from build123d import *

# Parameters (mm, degrees)
SKETCH_1_R          = 1.25
EXTRUDE_1_DEPTH     = 5
SKETCH_2_W          = 2.5
SKETCH_2_H          = 30.5
EXTRUDE_2_DEPTH     = 22.5
CUT_EXTRUDE_1_REACH = 107
SKETCH_4_R          = 3.5
SKETCH_4_R_2        = 1.25
SKETCH_4_W          = 30.5
SKETCH_4_H          = 14.5
EXTRUDE_3_DEPTH     = 2


with BuildPart() as part:
    # Эскиз1 → Бобышка-Вытянуть1 (new body)
    with BuildSketch(Plane(origin=(0, 0, 0), x_dir=(1, 0, 0), z_dir=(0, 1, 0))):
        with BuildLine():
            Line((-50, 32.5), (50, 32.5))
            ThreePointArc((50, 32.5), (51.767766953, 31.767766953), (52.5, 30))
            Line((52.5, 30), (52.5, -30))
            ThreePointArc((52.5, -30), (51.767766953, -31.767766953), (50, -32.5))
            Line((50, -32.5), (-50, -32.5))
            ThreePointArc((-50, -32.5), (-51.767766953, -31.767766953), (-52.5, -30))
            Line((-52.5, -30), (-52.5, -27.5))
            Line((-52.5, -27.5), (-52.5, 27.5))
            Line((-52.5, 27.5), (-52.5, 30))
            ThreePointArc((-52.5, 30), (-51.767766953, 31.767766953), (-50, 32.5))
        make_face()
        with Locations((-47.144457485, 27.207649218)):
            Circle(SKETCH_1_R, mode=Mode.SUBTRACT)
        with Locations((47.144457485, -27.207649218)):
            Circle(SKETCH_1_R, mode=Mode.SUBTRACT)
        with Locations((47.144457485, 27.207649218)):
            Circle(SKETCH_1_R, mode=Mode.SUBTRACT)
        with Locations((-47.144457485, -27.207649218)):
            Circle(SKETCH_1_R, mode=Mode.SUBTRACT)
        with BuildLine():
            Line((-40.944886513, 30), (40.944886513, 30))
            ThreePointArc((40.944886513, 30), (42.446070129, 29.321532349), (42.928749224, 27.74644775))
            ThreePointArc((42.928749224, 27.74644775), (44.154618836, 24.187158388), (47.726226395, 22.997655757))
            ThreePointArc((47.726226395, 22.997655757), (49.313859351, 22.524386076), (50, 21.016482364))
            Line((50, 21.016482364), (50, -21.016482364))
            ThreePointArc((50, -21.016482364), (49.313859351, -22.524386076), (47.726226395, -22.997655757))
            ThreePointArc((47.726226395, -22.997655757), (44.154618836, -24.187158388), (42.928749224, -27.74644775))
            ThreePointArc((42.928749224, -27.74644775), (42.446070129, -29.321532349), (40.944886513, -30))
            Line((40.944886513, -30), (-40.944886513, -30))
            ThreePointArc((-40.944886513, -30), (-42.446070129, -29.321532349), (-42.928749224, -27.74644775))
            ThreePointArc((-42.928749224, -27.74644775), (-44.154618836, -24.187158388), (-47.726226395, -22.997655757))
            ThreePointArc((-47.726226395, -22.997655757), (-49.313859351, -22.524386076), (-50, -21.016482364))
            Line((-50, -21.016482364), (-50, 21.016482364))
            ThreePointArc((-50, 21.016482364), (-49.313859351, 22.524386076), (-47.726226395, 22.997655757))
            ThreePointArc((-47.726226395, 22.997655757), (-44.154618836, 24.187158388), (-42.928749224, 27.74644775))
            ThreePointArc((-42.928749224, 27.74644775), (-42.446070129, 29.321532349), (-40.944886513, 30))
        make_face(mode=Mode.SUBTRACT)
    extrude(amount=EXTRUDE_1_DEPTH)

    # Эскиз2 → Бобышка-Вытянуть2 (add)
    with BuildSketch(Plane.XZ):
        with Locations((-51.25, 0)):
            Rectangle(SKETCH_2_W, SKETCH_2_H)
    extrude(amount=EXTRUDE_2_DEPTH)

    # Эскиз3 → Вырез-Вытянуть1 (cut, up to next)
    with BuildSketch(Plane.ZY.offset(52.5), mode=Mode.PRIVATE) as cut_extrude_1_sk1:
        with BuildLine():
            Line((-15.25, -22.5), (15.25, -22.5))
            ThreePointArc((15.25, -22.5), (0, -7.25), (-15.25, -22.5))
        make_face()
    cut_extrude_1_tool1 = extrude(cut_extrude_1_sk1.sketch, amount=-CUT_EXTRUDE_1_REACH, mode=Mode.PRIVATE) & part.part
    add(cut_extrude_1_tool1.solids().sort_by_distance((-52.5, -16.027699, 0))[0], mode=Mode.SUBTRACT)

    # Эскиз4 → Бобышка-Вытянуть3 (add)
    with BuildSketch(Plane(origin=(0, 5, 0), x_dir=(1, 0, 0), z_dir=(0, 1, 0))):
        with BuildLine():
            Line((-49.4756814, 32.562921498), (49.4756814, 32.562921498))
            ThreePointArc((49.4756814, 32.562921498), (51.597001743, 31.684241842), (52.4756814, 29.562921498))
            Line((52.4756814, 29.562921498), (52.4756814, -29.509131029))
            ThreePointArc((52.4756814, -29.509131029), (51.597001743, -31.630451373), (49.4756814, -32.509131029))
            Line((49.4756814, -32.509131029), (-49.4756814, -32.509131029))
            ThreePointArc((-49.4756814, -32.509131029), (-51.597001743, -31.630451373), (-52.4756814, -29.509131029))
            Line((-52.4756814, -29.509131029), (-52.4756814, 29.562921498))
            ThreePointArc((-52.4756814, 29.562921498), (-51.597001743, 31.684241842), (-49.4756814, 32.562921498))
        make_face()
        with Locations((26.75, -20)):
            Circle(SKETCH_4_R, mode=Mode.SUBTRACT)
        with Locations((-47.144457485, 27.207649218)):
            Circle(SKETCH_4_R_2, mode=Mode.SUBTRACT)
        with Locations((47.144457485, 27.207649218)):
            Circle(SKETCH_4_R_2, mode=Mode.SUBTRACT)
        with Locations((47.144457485, -27.207649218)):
            Circle(SKETCH_4_R_2, mode=Mode.SUBTRACT)
        with Locations((-47.144457485, -27.207649218)):
            Circle(SKETCH_4_R_2, mode=Mode.SUBTRACT)
        with Locations((26.75, 4.25)):
            Rectangle(SKETCH_4_W, SKETCH_4_H, mode=Mode.SUBTRACT)
    extrude(amount=EXTRUDE_3_DEPTH)


solid = part.part
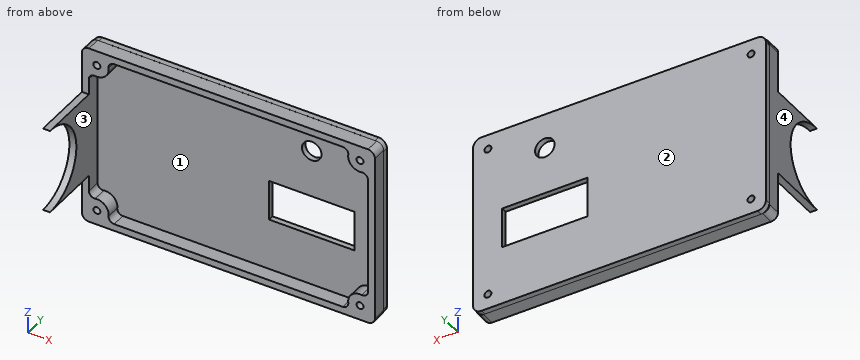
Source: CAD feature listing. Evaluate the final solid. Frame: model axes, mm. Face numbers are marked on the shaded views. A direction names the side the tool comes from. Give positions to 0.01 mm unless a question says otherwise; leave off trailing zeros. Write each loop counter-clockwise with the first axis right and the second up, starting at its lowest first coordinate (ties: lowest second). Pieces come first, ordered by that corner, then holes. Notation, with made-up numbers: M -16,28.25 L -4,28.25 A15 ccw -4,35.25 Z; hole C -25.5,-17 d5. An arc over 180 degrees is marked long. Return JSON: item names as keys, results as strings. Group by question number.
1) Set-up query: the marked faces 1 and 2. Return all of +Z, -Z, +X, -X, +Y, -Y with unobstructed straight access to the full face (end or side cutting, diameter ignored); none if empty.
2) First-contact query: pin 1 Ø2.5 at (x, y) = (10, 2.5) entering from -Z; pin 2 Ø1.6 at (y, z) = (6, 14) entering from -X; pin 3 Ø12 at (x, z) = (17, 15.5) entering from -Y; pin 4 Ø1.5 at (x, z) = (-47.14, 27.21) entering from -Y. Flat tips, straight axial feed; report the tip coordinate or a pass-through.
3) Cut plane C-C, the plane y = -11.25. Output: boundary loops of the cut face in (x, z), then the cut area to 3 significant figures.
4) Ray query, L1, parallel to Z at x = 14, y = 4.25; L2, parallel to X at y = 3.5, z = -17; L3, parallel to Y at x = -43.5, z = -19.5. Return the intervals inside material, ascending.
5) Draft query along Z for the marked faces 3 and 4. Return one class per face: released by +Z, released by -Z, zero draft, split by the parting line, or undercut.
Data:
{
 "1": {"face 1": "-Y", "face 2": "+Z, -Z, +X, -X, +Y"},
 "2": {"pin 1": "stops at z = -32.5", "pin 2": "stops at x = -52.48", "pin 3": "stops at y = 5", "pin 4": "passes through"},
 "3": {"outline": "M -52.5,-15.25 L -50,-15.25 L -50,-10.3 L -52.5,-10.3 Z; M -52.5,10.3 L -50,10.3 L -50,15.25 L -52.5,15.25 Z", "area": "24.8 mm²"},
 "4": {"L1": "z = -32.5 to -30, 30 to 32.5", "L2": "x = -52.5 to -50, 50 to 52.5", "L3": "y = 5 to 7"},
 "5": {"face 3": "undercut", "face 4": "zero draft"}
}
